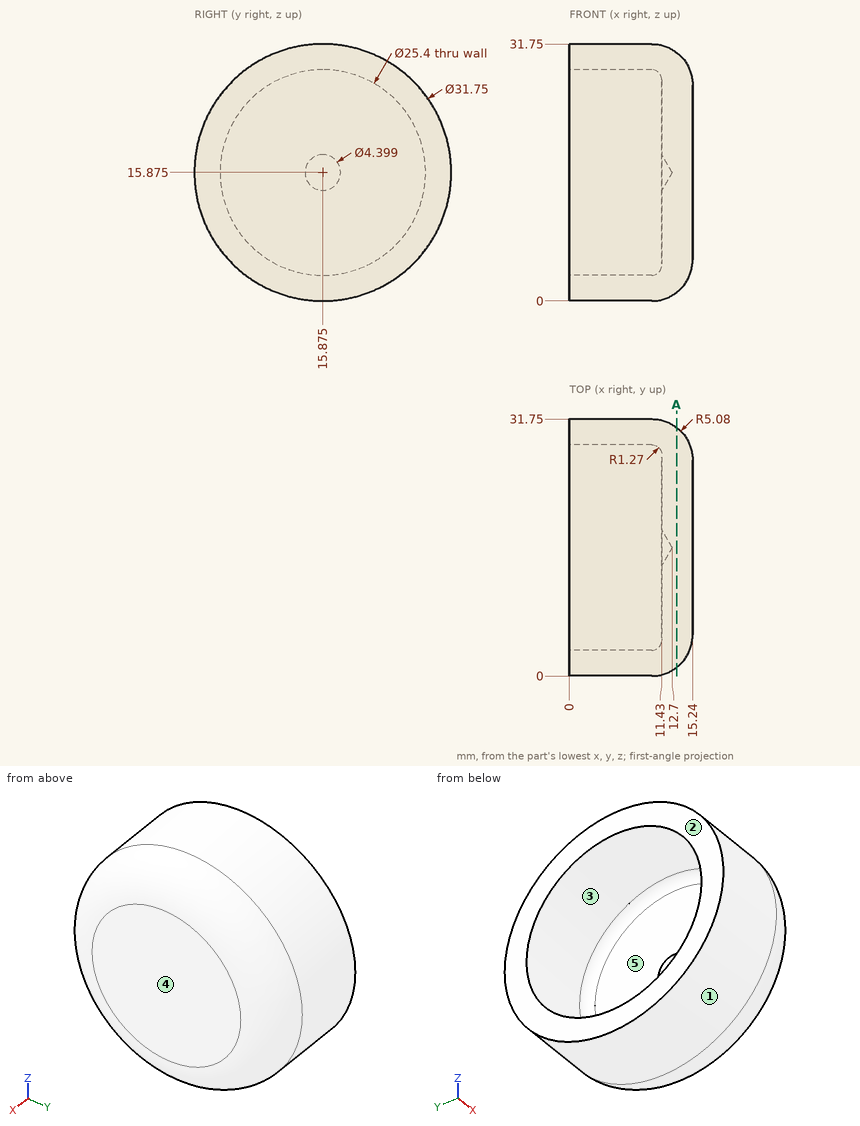
Check sheet for the drawn part. Datum: minimum x, y, z corner. Units: mm. A direction names the side the tool comes from. Give positions to 0.01 mm unless a question says otherwise; leave off trailing zeros. Order: outer loops, then holes, each group sorted by start corner. A loop starts at its lowest first (then second) coordinate and runs counter-clockwise, first axis right, second up. Notation, with made-up numbers: (64.5, -3.75) -> (75.5, -3.75) arc R27 cw to (75.5, 29.25) -> close; hole circle Ø4 at (85, 88.25). An arc over 180 degrees is marked (long way). Use a Markdown table: item, result.
1) Section check A-A, the plane x = 13.25. Record the boundary of the cut face in (y, z) (1 decimal).
Results:
| item | result |
|---|---|
| outline | circle Ø29.7 at (15.9, 15.9) |
2) Depth check by flat-ended pin: pin 1 Ø3 at (x, z) = (3, 6.5) entering from +Y; pin 2 Ø4 at (y, z) = (10, 10) entering from -X; pin 3 Ø4 at (x, z) = (3, 22.5) entering from +Y. Enter the tip coordinate at first touch or a pass-through.
Results:
| item | result |
|---|---|
| pin 1 | y = 29.66 |
| pin 2 | x = 11.43 |
| pin 3 | y = 31.06 |
3) Mould release check, pull along Z, two halves, no side actions. Record for the marked faces 1, 2 and 3: pulls with the +Z half, pulls with the -Z half, needs draft (parallel to the pull), parting line crosses it, or undercut.
Results:
| item | result |
|---|---|
| face 1 | parting line crosses it |
| face 2 | needs draft |
| face 3 | undercut |
4) Tool access check on the marked faces 4 and 5. Record the directions out of +Z, -Z, +X, -X, +Y, -Y that give a thin tool (end or side, any length) a straight path to the whole face; none if there is none.
Results:
| item | result |
|---|---|
| face 4 | +Z, -Z, +X, +Y, -Y |
| face 5 | -X |
5) Material ranges on probe 1 along Y at (x, z) = (9, 15.5) (1 decimal); probe 2 along Z at (x, y) = (1.5, 25) (1 decimal); probe 3 along X at (y, z) = (25, 11), recorded low to high.
Results:
| item | result |
|---|---|
| probe 1 | 0 to 3.2, 28.6 to 31.7 |
| probe 2 | 2.9 to 7, 24.7 to 28.9 |
| probe 3 | 11.43 to 15.24 |
